The drawing under review shows one solid part. Ordinate dimensions are in mm from its lowest x, y, z. A direction names the side the tool comes from. Round coordinates to 2 decimals unless told otherwise and drop trailing zeros. Order: outer loops, then holes, each group sorted by start corner. A loop starts at its lowest first (then second) coordinate and runs counter-clockwise, first axis right, second up. Notation, with made-up numbers: (43, 12) -> (53, 12) arc R6 cw to (53, 19) -> close; hole circle Ø11 at (82, 70). An arc over 180 degrees is marked (long way). Use a Markdown table: item, result. Add a question column.
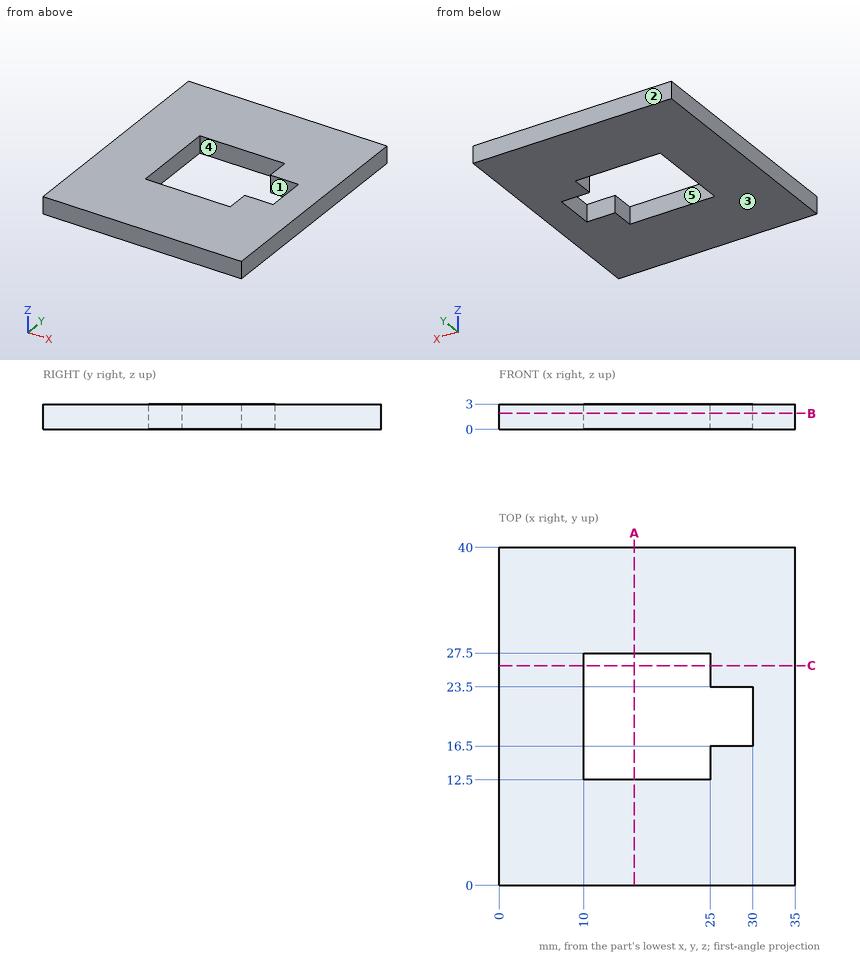
Q1. To check wall thickness, follow line 1 along X through (y, z) = (20.5, 0.7); line 2 along X through (y, z) = (16, 0.4); line 3 along Y through (x, z) = (10.5, 2.4). State the ranges of each line that lie inside material, in increasing order.
Q2. Add section B-B, the plane z = 1.9. Give the boundary of the cut face in (x, y), then the cut area to 3 significant figures.
Q3. For the marked faces 1 and 2, list the 3-axis set-ups (+Z, -Z, +X, -X, +Y, -Y) from which the entire face can be reached by the end or side of a thin tool; tool diameter is ignored.
Q4. Add section C-C, the plane y = 26. Give the boundary of the cut face in (x, z), then the cut area to 3 significant figures.
Q5. Add section A-A, the plane x = 16. Give the boundary of the cut face in (y, z).
Q6. Draft analysis for pull direction X (two halves, no side actions). For the marked faces 3, 4 and 5, state which applies: released by +X, released by -X, zero draft, split by the parting line, or undercut.
Return value:
| question | item | result |
|---|---|---|
| 1 | line 1 | 0 to 10, 30 to 35 |
| 1 | line 2 | 0 to 10, 25 to 35 |
| 1 | line 3 | 0 to 12.5, 27.5 to 40 |
| 2 | outline | (0, 0) -> (35, 0) -> (35, 40) -> (0, 40) -> close; hole (10, 12.5) -> (25, 12.5) -> (25, 16.5) -> (30, 16.5) -> (30, 23.5) -> (25, 23.5) -> (25, 27.5) -> (10, 27.5) -> close |
| 2 | area | 1,140 mm² |
| 3 | face 1 | +Z, -Z |
| 3 | face 2 | +Z, -Z, +X, -X, +Y |
| 4 | outline | (0, 0) -> (10, 0) -> (10, 3) -> (0, 3) -> close; (25, 0) -> (35, 0) -> (35, 3) -> (25, 3) -> close |
| 4 | area | 60.0 mm² |
| 5 | outline | (0, 0) -> (12.5, 0) -> (12.5, 3) -> (0, 3) -> close; (27.5, 0) -> (40, 0) -> (40, 3) -> (27.5, 3) -> close |
| 6 | face 3 | zero draft |
| 6 | face 4 | undercut |
| 6 | face 5 | undercut |
